For this review, use the dimensioned drawing (mm, ordinates from the lowest corner) and the shaded views. A direction names the side the tool comes from. Coordinates: 2 decimals unless noted, no trailing zeros. Order: outer loops, then holes, each group sorted by start corner. A loop starts at its lowest first (then second) coordinate and runs counter-clockwise, first axis right, second up. Notation, with made-up numbers: (49, -32.75) -> (107, -32.75) arc R13 cw to (107, -18.75) -> close; hole circle Ø11 at (76.5, 57). An arc over 180 degrees is marked (long way). Return JSON: item names as keys, results as strings. Group by question number.
Item 1: Machinability: for the marked faces 1, 2, 3 and 4, which of the approach directions +Z, -Z, +X, -X, +Y, -Y give a long, thin tool a straight path to every point of the face, cutting with its end or side? Answer none if there is none.
Item 2: Take a section at B-B (y = 2.5). Write out the cut boundary in (x, z), then the cut area to 3 significant figures.
Item 3: For line 1 along Y through (x, z) = (14, 10); line 2 along Z through (x, y) = (16.5, 2.25); line 3 along X through (y, z) = (9.25, 22), list the stretches that pass through material, from the lowest coordinate up.
Item 4: Insertion check: pin 1 (2 mm diameter, centred on x = 24.5, z = 32.5, fed in from -Y); pin 2 (1.4 mm diameter, centred on x = 21.5, y = 2.5, fed in from +Z); pin 3 (4 mm diameter, centred on x = 16, y = 11.5, fed in from -Z); pin 4 (4 mm diameter, centred on x = 8, y = 12.5, fed in from +Z). Each pin has a flat end and moves straight along its axis. Give the tip position at first contact, or say it passes through.
Item 5: Take a section at C-C (z = 17). Write out the cut boundary in (x, y), then the cut area to 3 significant figures.
Item 6: Take a section at A-A (x = 23). Write out the cut boundary in (y, z) (3 decimals), then the cut area to 3 significant figures.
Item 7: Take a section at D-D (z = 6). Write out the cut boundary in (x, y), then the cut area to 3 significant figures.
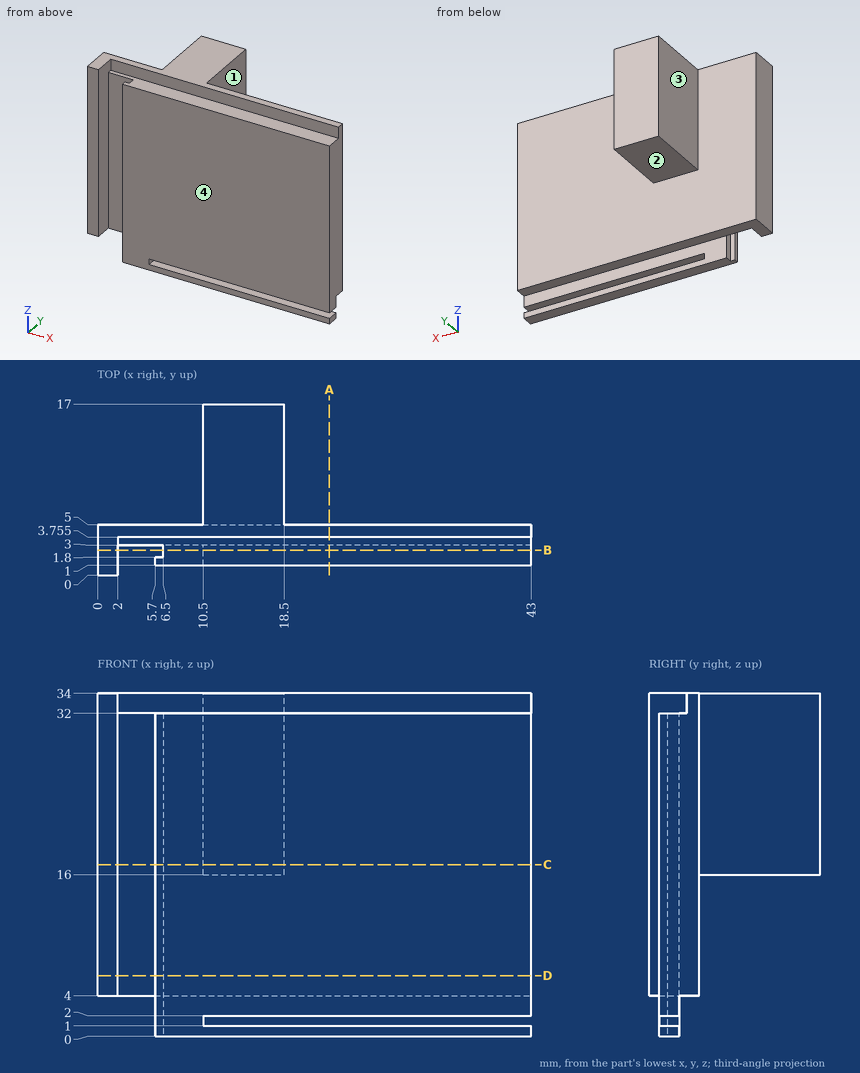
Findings below:
{
 "1": {"face 1": "+Z, -Z, +X, +Y", "face 2": "-Z, +X, -X, +Y", "face 3": "+Z, -Z, -X, +Y", "face 4": "+Z, -Z, +X, -Y"},
 "2": {"outline": "(0, 4) -> (2, 4) -> (2, 34) -> (0, 34) -> close; (6.5, 0) -> (43, 0) -> (43, 1) -> (10.5, 1) -> (10.5, 2) -> (43, 2) -> (43, 32) -> (6.5, 32) -> close", "area": "1,200 mm2"},
 "3": {"line 1": "y = 1 to 5", "line 2": "z = 0 to 1, 2 to 32", "line 3": "x = 10.5 to 18.5"},
 "4": {"pin 1": "stops at y = 1", "pin 2": "stops at z = 32", "pin 3": "stops at z = 16", "pin 4": "passes through"},
 "5": {"outline": "(0, 0) -> (2, 0) -> (2, 3) -> (6.5, 3) -> (6.5, 1.8) -> (5.7, 1.8) -> (5.7, 1) -> (43, 1) -> (43, 5) -> (18.5, 5) -> (18.5, 17) -> (10.5, 17) -> (10.5, 5) -> (0, 5) -> close", "area": "262 mm2"},
 "6": {"outline": "(1, 0) -> (3, 0) -> (3, 1) -> (1, 1) -> close; (1, 2) -> (3, 2) -> (3, 4) -> (5, 4) -> (5, 34) -> (3.755, 34) -> (3.755, 32) -> (1, 32) -> close", "area": "120 mm2"},
 "7": {"outline": "(0, 0) -> (2, 0) -> (2, 3) -> (6.5, 3) -> (6.5, 1.8) -> (5.7, 1.8) -> (5.7, 1) -> (43, 1) -> (43, 5) -> (0, 5) -> close", "area": "166 mm2"}
}
